The listing builds one solid part. Answer for the finished solid, in the listing's coordinates (mm). A direction names the side the tool comes from. Coordinates: 2 decimals unless noted, no trailing zeros. Loops run counter-clockwise (first coordinate to the right, second up) from the corner with the lowest first, then second, coordinate; pieces in that order, holes last. Notation, with made-up numbers: M 4,62 L 30,62 A27 ccw 30,89 Z; hole C -1.75,57.25 d10. An arc over 180 degrees is marked long. Return JSON: item names as keys, results as strings. Group by question number.
1. Which of the six approach directions +Z, -Z, +X, -X, +Y, -Y give full straight-line access (tool end or side, diameter ignored) to faces 1 (the face through (-3.22, 24.54, 38.2)), 2 (the face through (11, 1, 0)), 3 (the face through (3, 39, 15))?
2. The mould has two halves that part along X. Classify faces 4 (the face through (30.5, -12.6, 47.4)), 5 (the face through (30, 18, 30)), 6 (the face through (2, 26, 53.5)): pulls with the +X half, pulls with the -X half, needs draft (parallel to the pull), parting line crosses it, or undercut.
3. Straight lines are drawn through the part: L1, parallel to X at y = 17, z = 17; L2, parallel to Y at x = -32.5, z = 26; L3, parallel to Z at x = -16, y = 11. For each, find the intervals that lie inside material, in ascending order. Write a range as from..to.
4. Given P1, Ø25, axis at x = -5, y = 0.5, coming from the +Z side; P2, Ø3, axis at x = 32.5, y = -15.5, coming from the -Z side; P3, Ø12, axis at x = 7, z = 19, coming from the +Y side, each flat-ended and moving along its own axis, determine where each tip first touches the part or whether it passes through.
5. Section A-A (z = 45.5) is taken. Write down the section's boundary in (x, y).
6. Section B-B (z = 34) is taken. Write down the section's boundary in (x, y).
```python
from build123d import *

# Parameters (mm, degrees)
F0_R     = 51
F1_DEPTH = 42.5
F2_R     = 17.5
F3_R     = 5
F4_DEPTH = 30
F5_R     = 33
F6_DEPTH = 11
F7_R     = 1
F8_R     = 24.75
F9_DEPTH = 30
F10_R    = 1


with BuildPart() as f1:
    # F0 (on Top) → F1 (new body)
    with BuildSketch(Plane.XY):
        Circle(F0_R)
    extrude(amount=F1_DEPTH)

    # F2
    f2_edges = [f1.edges().sort_by_distance(p)[0] for p in [
        (-51, 0, 42.5),
    ]]
    fillet(f2_edges, radius=F2_R)

    # F3 (on Top) → F4 (cut)
    with BuildSketch(Plane.XY):
        with Locations((-30.3108891325, -17.5)):
            Circle(F3_R)
        with BuildLine():
            ThreePointArc((5, -35), (3.5355339059, -31.4644660941), (0, -30))
            ThreePointArc((0, -30), (-3.5355339059, -38.5355339059), (5, -35))
        make_face()
        with Locations((30.3108891325, -17.5)):
            Circle(F3_R)
        with Locations((30.3108891325, 17.5)):
            Circle(F3_R)
        with BuildLine():
            ThreePointArc((0, -5), (3.5355339059, -3.5355339059), (5, 0))
            ThreePointArc((5, 0), (-3.5355339059, 3.5355339059), (0, -5))
        make_face()
        with Locations((0, 35)):
            Circle(F3_R)
        with Locations((-30.3108891325, 17.5)):
            Circle(F3_R)
    extrude(amount=F4_DEPTH, mode=Mode.SUBTRACT)

    # F5 (on face) → F6 (join)
    with BuildSketch(Plane.XY.offset(42.5)):
        Circle(F5_R)
    extrude(amount=F6_DEPTH)

    # F7
    f7_edges = [f1.edges().sort_by_distance(p)[0] for p in [
        (-33, 0, 53.5),
    ]]
    fillet(f7_edges, radius=F7_R)

    # F8 (on face) → F9 (cut)
    with BuildSketch(Plane.XY.offset(53.5)):
        Circle(F8_R)
    extrude(amount=-F9_DEPTH, mode=Mode.SUBTRACT)

    # F10
    f10_edges = [f1.edges().sort_by_distance(p)[0] for p in [
        (-32, 0, 53.5),
        (-24.75, 0, 53.5),
    ]]
    fillet(f10_edges, radius=F10_R)


solid = f1.part
```
Worked out:
{
 "1": {"face 1": "+Z", "face 2": "-Z, +X, -X, +Y, -Y", "face 3": "-Z"},
 "2": {"face 4": "parting line crosses it", "face 5": "undercut", "face 6": "needs draft"},
 "3": {"L1": "-48.08..-35.29, -25.34..25.34, 35.29..48.08", "L2": "-39.27..-22, -13..13, 22..39.27", "L3": "0..23.5"},
 "4": {"P1": "z = 23.5", "P2": "z = 30", "P3": "y = 50.99"},
 "5": {"outline": "C 0,0 d66; hole C 0,0 d49.5"},
 "6": {"outline": "C 0,0 d97.02; hole C 0,0 d49.5"}
}
